```python
from build123d import *

# Parameters (mm, degrees)
BOSS_EXTRUDE1_DEPTH      = 2.54
CUT_EXTRUDE1_DEPTH       = 3.54
BOSS_EXTRUDE2_DEPTH      = 25.4
BOSS_EXTRUDE2_DEPTH_BACK = 25.4
BOSS_EXTRUDE3_DEPTH      = 30.48
CUT_EXTRUDE2_DEPTH       = 19.05
CHAMFER2_SIZE            = 5.08
BOSS_EXTRUDE4_DEPTH      = 33.02


with BuildPart() as part:
    # Sketch1 → Boss-Extrude1 (new body)
    with BuildSketch(Plane(origin=(0, 0, 0), x_dir=(1, 0, 0), z_dir=(0, 1, 0))):
        Polygon((-36.195, 66.167), (36.195, 66.167), (60.706, 41.656), (60.706, -41.656), (36.195, -66.167), (-36.195, -66.167), (-60.706, -41.656), (-60.706, 41.656), align=None)
    extrude(amount=BOSS_EXTRUDE1_DEPTH)

    # Sketch5 → Cut-Extrude1 (cut, through all)
    with BuildSketch(Plane(origin=(0, 2.54, 0), x_dir=(1, 0, 0), z_dir=(0, 1, 0))):
        Polygon((58.166, -44.196), (36.195, -66.167), (17.145, -66.167), (39.116, -44.196), align=None)
    extrude(amount=-CUT_EXTRUDE1_DEPTH, mode=Mode.SUBTRACT)

    # Sketch3 → Boss-Extrude2 (add, two sides)
    with BuildSketch(Plane.XY) as boss_extrude2_sk:
        Polygon((-53.848, 2.54), (-57.658, 6.35), (-54.065897552, 6.35), (-50.255897552, 2.54), align=None)
        Polygon((54.065897552, 6.35), (50.255897552, 2.54), (53.848, 2.54), (57.658, 6.35), align=None)
    extrude(amount=BOSS_EXTRUDE2_DEPTH)
    extrude(boss_extrude2_sk.sketch, amount=-BOSS_EXTRUDE2_DEPTH_BACK)

    # Sketch4 → Boss-Extrude3 (add)
    with BuildSketch(Plane(origin=(0, 2.54, 0), x_dir=(1, 0, 0), z_dir=(0, 1, 0))):
        Polygon((60.706, -41.656), (58.166, -41.656), (38.063897552, -41.656), (16.092897552, -63.627), (-35.142897552, -63.627), (-57.113897552, -41.656), (-60.706, -41.656), (-36.195, -66.167), (17.145, -66.167), (39.116, -44.196), (58.166, -44.196), align=None)
    extrude(amount=BOSS_EXTRUDE3_DEPTH)

    # Sketch6 → Cut-Extrude2 (cut)
    with BuildSketch(Plane(origin=(0, 33.02, 0), x_dir=(1, 0, 0), z_dir=(0, 1, 0))):
        Polygon((38.063897552, -41.656), (16.092897552, -63.627), (17.145, -66.167), (39.116, -44.196), align=None)
    extrude(amount=-CUT_EXTRUDE2_DEPTH, mode=Mode.SUBTRACT)

    # Chamfer2
    chamfer2_edges = [part.edges().sort_by_distance(p)[0] for p in [
        (16.618948776, 13.97, 64.897),
        (38.589948776, 13.97, 42.926),
    ]]
    chamfer(chamfer2_edges, length=CHAMFER2_SIZE)

    # Sketch7 → Boss-Extrude4 (add)
    with BuildSketch(Plane.XZ):
        Polygon((-8.255, 66.167), (-8.255, 71.247), (-10.795, 71.247), (-15.875, 66.167), align=None)
        Polygon((10.795, 71.247), (15.875, 66.167), (8.255, 66.167), (8.255, 71.247), align=None)
    extrude(amount=-BOSS_EXTRUDE4_DEPTH)


solid = part.part
```
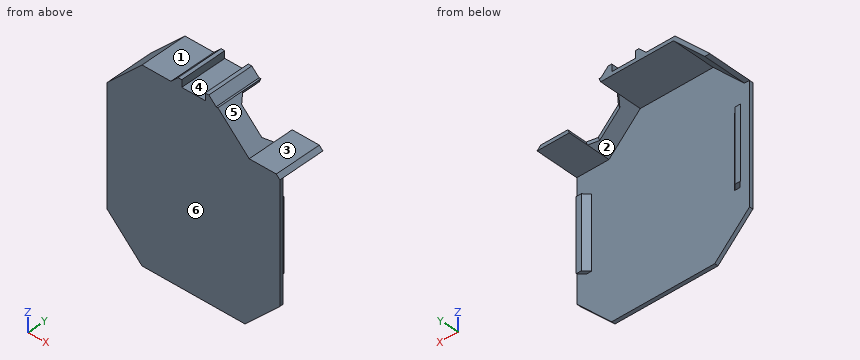
Could you check a few things on this model? Use its own coordinates, in mm. Face numbers are marked on the shaded views. A direction names the side the tool comes from. Round coordinates to 2 decimals unless told otherwise and drop trailing zeros. Write each loop counter-clockwise with the first axis right and the second up, starting at its lowest first coordinate (ties: lowest second). Pieces come first, ordered by that corner, then holes. Notation, with made-up numbers: M 12.25,-26.75 L 71.25,-26.75 A34 cw 71.25,6.25 Z; hole C 17,29.25 d7. An arc over 180 degrees is marked long. Write each question's results on one line, items separated by ' | '. Start each with the question number.
1. Imagine slicing it at A-A on y = 25. List the corners of the cut face in (x, z) for me (3 decimals), and give its area (3 significant figures).
2. Imagine slicing it at D-D on x = -19. List the corners of the cut face in (y, z) for me.
3. I'm going to push flat-ended pins straight in: pin 1 Ø3 at (x, y) = (12, 25) entering from -Z; pin 2 Ø1.8 at (x, z) = (56, 11) entering from +Y; pin 3 Ø4 at (y, z) = (20, 68.5) entering from +X; pin 4 Ø5 at (y, z) = (21.5, 38.5) entering from -X. Where does each tip first touch, or does it pass through?
4. Imagine slicing it at C-C on z = 8. List the corners of the cut face in (x, y) for me.
5. Imagine slicing it at B-B on y = 10. List the corners of the cut face in (x, z) for me (3 decimals), and give its area (3 significant figures).
6. On a 3-axis mill with a long thin cutter (end or side, diameter ignored), from which of +Z, -Z, +X, -X, +Y, -Y can I reach the whole of each face in a straight line? I mean the marked faces 1, 2 and 3. Say none if no direction works.
7. I need wall thicknesses on L1, parallel to Z at x = 47, y = 7.5; L2, parallel to Y at x = -48, z = -24; L3, parallel to Z at x = 6, y = 17.5. Which ranges of each line are inside material? Lowest first, please. Write a range as from..to.
8. Thinking about a two-plate mould opening in X: for the marked faces 4, 5 and 6, which applies, +X half, -X half, draft (parallel to the pull), parting line (faces both ways), or undercut?
Result sheet:
1) outline: M -60.706,41.656 L -57.114,41.656 L -35.143,63.627 L 16.093,63.627 L 17.145,66.167 L 15.875,66.167 L 10.795,71.247 L 8.255,71.247 L 8.255,66.167 L -8.255,66.167 L -8.255,71.247 L -10.795,71.247 L -15.875,66.167 L -36.195,66.167 Z; M 38.064,41.656 L 60.706,41.656 L 58.166,44.196 L 39.116,44.196 Z | area: 321 mm^2
2) outline: M 0,-66.17 L 2.54,-66.17 L 2.54,63.63 L 33.02,63.63 L 33.02,66.17 L 0,66.17 Z
3) pin 1: stops at z = 63.63 | pin 2: stops at y = 6.35 | pin 3: stops at x = 15.54 | pin 4: passes through
4) outline: M -60.71,0 L 60.71,0 L 60.71,2.54 L 53.85,2.54 L 57.66,6.35 L 54.07,6.35 L 50.26,2.54 L -50.26,2.54 L -54.07,6.35 L -57.66,6.35 L -53.85,2.54 L -60.71,2.54 Z
5) outline: M -60.706,41.656 L -57.114,41.656 L -35.143,63.627 L 16.093,63.627 L 38.064,41.656 L 60.706,41.656 L 58.166,44.196 L 39.116,44.196 L 17.145,66.167 L 15.875,66.167 L 10.795,71.247 L 8.255,71.247 L 8.255,66.167 L -8.255,66.167 L -8.255,71.247 L -10.795,71.247 L -15.875,66.167 L -36.195,66.167 Z | area: 400 mm^2
6) face 1: +Z, -X, +Y, -Y | face 2: -Z, +Y | face 3: +Z, +X, +Y, -Y
7) L1: z = 41.66..44.2 | L2: y = 0..2.54 | L3: z = 63.63..66.17
8) face 4: undercut | face 5: +X half | face 6: draft
